Can you work these out from the drawing? Everything is in mm from the part's minimum corner. Coordinates: 2 decimals unless noted, no trailing zeros. Loops run counter-clockwise (first coordinate to the right, second up) from the corner with the lowest first, then second, coordinate; pieces in that order, holes last. Notation, with made-up numbers: (77, 83.5) -> (102, 83.5) arc R12 ccw to (102, 87.5) -> close; hole circle Ø6 at (33.5, 32.25). An arc over 180 degrees is marked (long way). Use one line per item in the form item = value. Start each with the question number.
(1) Imagine slicing it at C-C (x = 69). List the corners of the cut face in (y, z) for me.
(2) Imagine slicing it at A-A (z = 34). List the corners of the cut face in (x, y) for me, plus the area to 3 significant figures.
(3) I'm going to push a flat-ended pin straight in: pin 1 (2.5 mm diameter, centred on x = 29, z = 50, fed in from +Y). Where does the tip first touch, or does it pass through?
(4) I need wall thicknesses on line 1 (X direction, y = 2.15, z = 10); line 2 (X direction, y = 3.95, z = 74); line 3 (Z direction, x = 69, y = 2.7). Which ranges of each line are inside material? Lowest first, please. Write a range as [from, to].
(5) Imagine slicing it at B-B (y = 2.8). State how many separate pieces and enclosed holes the cut face has, plus the area to 3 significant figures.
(6) Imagine slicing it at D-D (z = 74). List the corners of the cut face in (x, y) for me.
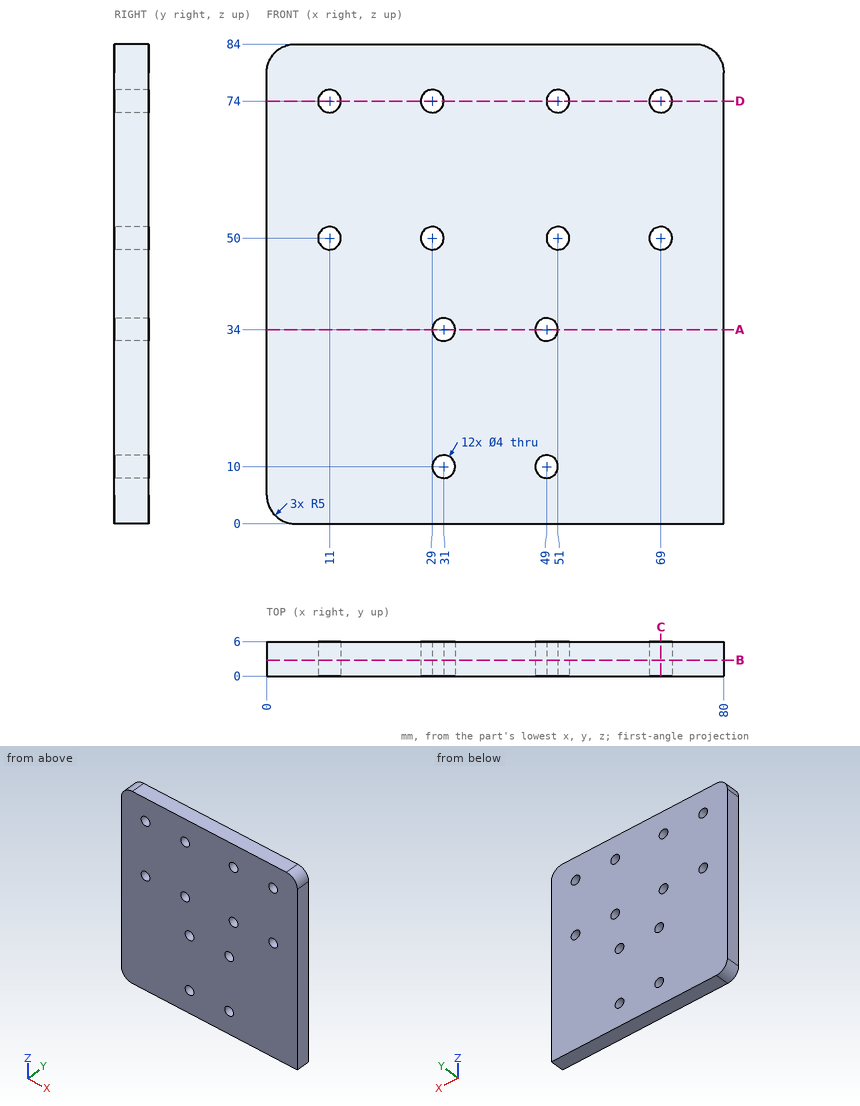
Worked out:
q1.outline = (0, 0) -> (6, 0) -> (6, 48) -> (0, 48) -> close; (0, 52) -> (6, 52) -> (6, 72) -> (0, 72) -> close; (0, 76) -> (6, 76) -> (6, 84) -> (0, 84) -> close
q2.outline = (0, 0) -> (29, 0) -> (29, 6) -> (0, 6) -> close; (33, 0) -> (47, 0) -> (47, 6) -> (33, 6) -> close; (51, 0) -> (80, 0) -> (80, 6) -> (51, 6) -> close
q2.area = 432 mm2
q3.pin_1 = through
q4.line_1 = [0, 29], [33, 47], [51, 80]
q4.line_2 = [0, 9], [13, 27], [31, 49], [53, 67], [71, 80]
q4.line_3 = [0, 48], [52, 72], [76, 84]
q5.separate_pieces = 1
q5.enclosed_holes = 12
q5.area = 6,550 mm2
q6.outline = (0, 0) -> (9, 0) -> (9, 6) -> (0, 6) -> close; (13, 0) -> (27, 0) -> (27, 6) -> (13, 6) -> close; (31, 0) -> (49, 0) -> (49, 6) -> (31, 6) -> close; (53, 0) -> (67, 0) -> (67, 6) -> (53, 6) -> close; (71, 0) -> (80, 0) -> (80, 6) -> (71, 6) -> close
